Source: CAD feature listing. Evaluate the final solid. Frame: model axes, mm. Round coordinates to 2 decimals unless told otherwise and drop trailing zeros. Order: outer loops, then holes, each group sorted by start corner. A loop starts at its lowest first (then second) coordinate and runs counter-clockwise, first axis right, second up. Notation, with made-up numbers: (-31.5, 24.25) - (22.5, 24.25) arc R20 ccw to (22.5, 33.25) - close; hole circle Ø10 at (80.5, -1.75). An arc over 180 degrees is marked (long way). Put each result on its own line as item: value. Start each with the question number.
1) Contact query for flat-ended pins moving along their axis: P1, Ø3, axis at x = 0, y = 0, coming from the +Z side; P2, Ø1.5, axis at x = -2, z = -0.5, coming from the +Y side. Output: stop coordinate, or through.
2) Section C-C on x = -4.5. Output: boundary loops of the cut face in (y, z).
3) Mould query, pull axis X, two halves, no side actions, for faces 1 (the face through (0.16, -67.5, 0.02)), 2 (the face through (0, 2, 0)), 3 (the face through (7.5, -30, 0)). Classes: +X half, -X half, draft (parallel to the pull), parting line (faces both ways), or undercut.
4) Section B-B on z = -0.85. Output: boundary loops of the cut face in (x, y) (3 decimals), then the cut area to 3 significant figures.
5) Section A-A on x = 0. Output: boundary loops of the cut face in (y, z) (3 decimals), then the cut area to 3 significant figures.
6) Line query: probe 1 along Y at (x, z) = (0, 0.6) (3 decimals); probe 2 along Y at (x, z) = (-2.25, -0.25); probe 3 along X at (y, z) = (-2, -1.1). Output: solid intervals per line, ascending. Write a range as [from, to].
```python
from build123d import *

# Parameters (mm, degrees)
CROQUIS1_R                   = 3.175
SALIENTE_EXTRUIR1_DEPTH      = 1.5
SALIENTE_EXTRUIR1_DEPTH_BACK = 1.5


with BuildPart() as part:
    # Croquis1 → Saliente-Extruir1 (new body, two sides)
    with BuildSketch(Plane.XY) as saliente_extruir1_sk:
        with BuildLine():
            Line((7.5, 0), (7.5, -60))
            ThreePointArc((7.5, -60), (0, -67.5), (-7.5, -60))
            Line((-7.5, -60), (-7.5, 0))
            ThreePointArc((-7.5, 0), (0, 7.5), (7.5, 0))
        make_face()
        with Locations((0, -60)):
            Circle(CROQUIS1_R, mode=Mode.SUBTRACT)
        with BuildLine():
            Line((-1.5, 2), (1.5, 2))
            ThreePointArc((1.5, 2), (0, -2.5), (-1.5, 2))
        make_face(mode=Mode.SUBTRACT)
    extrude(amount=SALIENTE_EXTRUIR1_DEPTH)
    extrude(saliente_extruir1_sk.sketch, amount=-SALIENTE_EXTRUIR1_DEPTH_BACK)


solid = part.part
```
Answer sheet:
1. P1: through
1. P2: y = 7.4
2. outline: (-66, -1.5) - (6, -1.5) - (6, 1.5) - (-66, 1.5) - close
3. face 1: parting line
3. face 2: undercut
3. face 3: +X half
4. outline: (-7.5, -60) arc R7.5 ccw to (7.5, -60) - (7.5, 0) arc R7.5 ccw to (-7.5, 0) - close; hole circle Ø6.35 at (0, -60); hole (-1.5, 2) arc R2.5 ccw (long way) to (1.5, 2) - close
4. area: 1,030 mm^2
5. outline: (-67.5, -1.5) - (-63.175, -1.5) - (-63.175, 1.5) - (-67.5, 1.5) - close; (-56.825, -1.5) - (-2.5, -1.5) - (-2.5, 1.5) - (-56.825, 1.5) - close; (2, -1.5) - (7.5, -1.5) - (7.5, 1.5) - (2, 1.5) - close
5. area: 192 mm^2
6. probe 1: [-67.5, -63.175], [-56.825, -2.5], [2, 7.5]
6. probe 2: [-67.15, -62.24], [-57.76, -1.09], [1.09, 7.15]
6. probe 3: [-7.5, -1.5], [1.5, 7.5]
